```python
from build123d import *

# Parameters (mm, degrees)
SKETCH1_R           = 4
EXTRUDE1_DEPTH      = 2.6
EXTRUDE2_START      = -4
EXTRUDE2_DEPTH      = 5
CUT_EXTRUDE1_DEPTH  = 0.2
SKETCH12_R          = 1.5
BOSS_EXTRUDE3_DEPTH = 0.15
FILLET4_R           = 0.05
EXTRUDE_THIN1_START = 1.1
EXTRUDE_THIN1_DEPTH = 0.4
EXTRUDE3_DEPTH      = 0.25
SKETCH10_R          = 3
EXTRUDE6_DEPTH      = 0.25
SKETCH13_W          = 0.5
SKETCH13_H          = 2.199959577
BOSS_EXTRUDE4_DEPTH = 0.25
CIRPATTERN1_COUNT   = 2


with BuildPart() as part:
    # Sketch1 → Extrude1 (new body)
    with BuildSketch(Plane(origin=(0, 0, 0), x_dir=(1, 0, 0), z_dir=(0, 1, 0))):
        with Locations(Location((0, 0, 0), (0, 0, 270))):
            Circle(SKETCH1_R)
    extrude(amount=EXTRUDE1_DEPTH)

    # Extrude2: read off the stored shape, not the designer's step
    # Extrude2 outline → Extrude2 (cut)
    with BuildSketch(Plane(origin=(0, 2.6, 0), x_dir=(1, 0, 0), z_dir=(0, 1, 0)).offset(EXTRUDE2_START)):
        with BuildLine():
            Line((-3.6, -1.743559577), (-3.6, 1.743559577))
            ThreePointArc((-3.6, 1.743559577), (-4, 0), (-3.6, -1.743559577))
        make_face()
        with BuildLine():
            ThreePointArc((3.6, -1.743559577), (4, 0), (3.6, 1.743559577))
            Line((3.6, 1.743559577), (3.6, -1.743559577))
        make_face()
    extrude(amount=EXTRUDE2_DEPTH, mode=Mode.SUBTRACT)

    # Sketch2<3> → Cut-Extrude1 (cut)
    with BuildSketch(Plane(origin=(0, 2.6, 0), x_dir=(1, 0, 0), z_dir=(0, 1, 0))):
        with BuildLine():
            ThreePointArc((-0.596992462, -2.94), (0, -3.6), (0.596992462, -2.94))
            ThreePointArc((0.596992462, -2.94), (3, 0), (0.596992462, 2.94))
            ThreePointArc((0.596992462, 2.94), (0, 3.6), (-0.596992462, 2.94))
            ThreePointArc((-0.596992462, 2.94), (-3, 0), (-0.596992462, -2.94))
        make_face()
    extrude(amount=-CUT_EXTRUDE1_DEPTH, mode=Mode.SUBTRACT)

    # Sketch12 → Boss-Extrude3 (add)
    with BuildSketch(Plane(origin=(0, 2.4, 0), x_dir=(1, 0, 0), z_dir=(0, 1, 0))):
        with Locations(Location((0, 0, 0), (0, 0, 270))):
            Circle(SKETCH12_R)
    extrude(amount=BOSS_EXTRUDE3_DEPTH)

    # Fillet4
    fillet4_edges = [part.edges().sort_by_distance(p)[0] for p in [
        (0, 2.55, -1.5),
    ]]
    fillet(fillet4_edges, radius=FILLET4_R)

    # Sketch6 → Extrude-Thin1 (add, symmetric)
    with BuildSketch(Plane.XY.offset(EXTRUDE_THIN1_START)):
        with BuildLine():
            Line((-3.6, 1.3), (-4.416697321, 1.3))
            ThreePointArc((-4.416697321, 1.3), (-4.721601087, 1.19627477), (-4.9, 0.928134773))
            Line((-4.9, 0.928134773), (-5.047479985, 0.371865227))
            ThreePointArc((-5.047479985, 0.371865227), (-5.225878898, 0.10372523), (-5.530782665, 0))
            Line((-5.530782665, 0), (-7.25, 0))
            Line((-7.25, 0), (-7.25, 0.25))
            Line((-7.25, 0.25), (-5.530782665, 0.25))
            ThreePointArc((-5.530782665, 0.25), (-5.378330782, 0.301862615), (-5.289131325, 0.435932613))
            Line((-5.289131325, 0.435932613), (-5.14165134, 0.99220216))
            ThreePointArc((-5.14165134, 0.99220216), (-4.87405297, 1.394412155), (-4.416697321, 1.55))
            Line((-4.416697321, 1.55), (-3.6, 1.55))
            Line((-3.6, 1.55), (-3.6, 1.3))
        make_face()
    extrude_thin1 = extrude(amount=EXTRUDE_THIN1_DEPTH, both=True)

    # Sketch7 → Extrude3 (add)
    with BuildSketch(Plane(origin=(0, 0.25, 0), x_dir=(1, 0, 0), z_dir=(0, 1, 0))):
        Polygon((-5.9, -0.7), (-6.25, -0.35), (-7.25, -0.35), (-7.25, -1.85), (-6.25, -1.85), (-5.9, -1.5), align=None)
    extrude3 = extrude(amount=-EXTRUDE3_DEPTH)

    # Sketch10 → Extrude6 (cut)
    with BuildSketch(Plane.XZ):
        with BuildLine():
            Line((3.6, -1.743559577), (3.6, 1.743559577))
            ThreePointArc((3.6, 1.743559577), (0, 4), (-3.6, 1.743559577))
            Line((-3.6, 1.743559577), (-3.6, -1.743559577))
            ThreePointArc((-3.6, -1.743559577), (0, -4), (3.6, -1.743559577))
        make_face()
        with Locations(Location((0, 0, 0), (0, 0, 270))):
            Circle(SKETCH10_R, mode=Mode.SUBTRACT)
    extrude(amount=-EXTRUDE6_DEPTH, mode=Mode.SUBTRACT)

    # Sketch13 → Boss-Extrude4 (add)
    with BuildSketch(Plane(origin=(0, 1.55, 0), x_dir=(1, 0, 0), z_dir=(0, 1, 0))):
        with Locations((-3.85, 0.399979788)):
            Rectangle(SKETCH13_W, SKETCH13_H)
    boss_extrude4 = extrude(amount=-BOSS_EXTRUDE4_DEPTH)

    # CirPattern1: Extrude-Thin1, Extrude3, Boss-Extrude4 ×2 about axis
    cirpattern1_axis = Axis((0, 0, 0), (0, 1, 0))
    add([extrude_thin1.rotate(cirpattern1_axis, i * 360 / CIRPATTERN1_COUNT) for i in range(1, CIRPATTERN1_COUNT)])
    add([extrude3.rotate(cirpattern1_axis, i * 360 / CIRPATTERN1_COUNT) for i in range(1, CIRPATTERN1_COUNT)])
    add([boss_extrude4.rotate(cirpattern1_axis, i * 360 / CIRPATTERN1_COUNT) for i in range(1, CIRPATTERN1_COUNT)])


solid = part.part
```
Check sheet for the modelled part. Datum: model origin and axes. Units: mm. A direction names the side the tool comes from. Round coordinates to 2 decimals unless told otherwise and drop trailing zeros. Loops run counter-clockwise (first coordinate to the right, second up) from the corner with the lowest first, then second, coordinate; pieces in that order, holes last. Notation, with made-up numbers: (2, 89.25) - (41, 89.25) arc R9 ccw to (41, 93.25) - close; hole circle Ø6 at (-8.5, 22). An arc over 180 degrees is marked (long way). Write item = value, one per line. Start each with the question number.
Q1. Section check C-C (z = 2.5). Record the boundary of the cut face in (x, y).
Q2. Depth check by flat-ended pin: P1, Ø0.8, axis at x = -6.5, z = 1, coming from the +Y side; P2, Ø0.7, axis at x = 4, z = -0.5, coming from the -Y side; P3, Ø1, axis at x = -4, z = 2.5, coming from the +Y side; P4, Ø0.5, axis at x = -5, y = 0.5, coming from the +Z side. Enter the tip coordinate at first touch or a pass-through.
Q3. Thickness scan on L1, parallel to Y at x = 1.75, z = -2.5; L2, parallel to Y at x = 0, z = -0.75; L3, parallel to X at y = 2.55, z = 3. Record the ranges inside material, lowest first.
Q4. Release check for a two-part mould opening along Z. For faces 4 (the face through (-1.4, 2.4, -0.9)), 5 (the face through (3.9, 1.3, -0.3)) record: pulls with the +Z half, pulls with the -Z half, needs draft (parallel to the pull), parting line crosses it, or undercut.
Q5. Section check A-A (z = 0). Record the boundary of the cut face in (x, y), plus the area to 3 significant figures.
Q6. Access from +Z, -Z, +X, -X, +Y, -Y to the whole of each face (thin tool, end or side, straight path). Record for faces 1 (the face through (6, 0.25, -1)), 2 (the face through (-3.9, 1.55, 0.3)), 3 (the face through (-1, 0.25, -3)).
Q7. Section check B-B (y = 2). Record the boundary of the cut face in (x, z).
Derived:
q1.outline = (-3.12, 0.25) - (-1.66, 0.25) - (-1.66, 0) - (1.66, 0) - (1.66, 0.25) - (3.12, 0.25) - (3.12, 2.6) - (1.66, 2.6) - (1.66, 2.4) - (-1.66, 2.4) - (-1.66, 2.6) - (-3.12, 2.6) - close
q2.P1 = 0.25
q2.P2 = 1.3
q2.P3 = through
q2.P4 = 1.5
q3.L1 = 0.25 to 2.6
q3.L2 = 0 to 2.55
q3.L3 = -2.65 to -0.6, 0.6 to 2.65
q4.face_4 = undercut
q4.face_5 = needs draft
q5.outline = (-4.1, 1.3) - (-3.6, 1.3) - (-3.6, 0.25) - (-3, 0.25) - (-3, 0) - (3, 0) - (3, 0.25) - (3.6, 0.25) - (3.6, 1.3) - (4.1, 1.3) - (4.1, 1.55) - (3.6, 1.55) - (3.6, 2.6) - (3, 2.6) - (3, 2.4) - (1.5, 2.4) - (1.5, 2.5) arc R0.05 ccw to (1.45, 2.55) - (-1.45, 2.55) arc R0.05 ccw to (-1.5, 2.5) - (-1.5, 2.4) - (-3, 2.4) - (-3, 2.6) - (-3.6, 2.6) - (-3.6, 1.55) - (-4.1, 1.55) - close
q5.area = 17.9 mm^2
q6.face_1 = +Z, -Z, +X, +Y
q6.face_2 = +Z, -Z, -X, +Y
q6.face_3 = -Y
q7.outline = (-3.6, -1.74) arc R4 ccw to (3.6, -1.74) - (3.6, 1.74) arc R4 ccw to (-3.6, 1.74) - close
